CAD build for the part. Positions are in the model's coordinates, mm. A direction names the side the tool comes from. Give positions to 0.01 mm unless a question says otherwise; leave off trailing zeros. Write each loop counter-clockwise with the first axis right and the second up, starting at its lowest first coordinate (ties: lowest second). Pieces come first, ordered by that corner, then holes. Notation, with made-up numbers: (79.25, -39.75) -> (121.25, -39.75) arc R17 cw to (121.25, -34.75) -> close; hole circle Ø4 at (12.25, -4.75). An arc over 180 degrees is marked (long way). Answer as a JSON object with one key per item and string values.
```python
from build123d import *

# Parameters (mm, degrees)
F1_DEPTH  = 20
F3_R      = 3.5
F4_DEPTH  = 10
F8_R      = 3.5
F9_DEPTH  = 1
F9_FACE_R = 3.5


with BuildPart() as f1:
    # F0 (on Front) → F1 (new body)
    with BuildSketch(Plane.XZ):
        Polygon((0, -40), (0, 0), (60, 0), (60, 5), (-5, 5), (-5, -45), (40, -45), (40, -40), align=None)
    extrude(amount=F1_DEPTH)

    # F3 (on offset) → F4 (join)
    with BuildSketch(Plane(origin=(0, 0, -45), x_dir=(1, 0, 0), z_dir=(0, 0, -1))):
        with Locations((33.4731638432, 10)):
            Circle(F3_R)
    extrude(amount=F4_DEPTH)



with BuildPart() as f9:
    # F8 (on offset) → F9 (new body)
    with BuildSketch(Plane(origin=(0, 0, -55), x_dir=(1, 0, 0), z_dir=(0, 0, -1))):
        with Locations((13.4731638432, 10)):
            Circle(F8_R)
    extrude(amount=-F9_DEPTH)


with BuildPart() as f1_1:
    add(f1.part)

    add(f9.part)  # F10 merges F9
    # F10: sweep along a path in F6
    with BuildLine(Plane(origin=(0, -10, 0), x_dir=(-1, 0, 0), z_dir=(0, 1, 0))) as f10_path:
        ThreePointArc((-33.4731638432, -55), (-23.4731638432, -65), (-13.4731638432, -55))
    # F9_face (on face) → F10 (sweep)
    with BuildSketch(Plane(origin=(13.4731638432, -10, -55), x_dir=(1, 0, 0), z_dir=(0, 0, -1))):
        Circle(F9_FACE_R)
    sweep(path=f10_path.line)


solid = f1_1.part
```
1) Slice it at C-C (z = -38.5). List the corners of the cut face in (x, y).
Model answer:
{"outline": "(-5, -20) -> (0, -20) -> (0, 0) -> (-5, 0) -> close"}
2) Pin check, flat tip, straight feed: pin 1 (2.5 mm diameter, centred on y = -9, z = -41.5, fed in from +X). Stop position of the tip, or through.
Model answer:
{"pin 1": "stops at x = 40"}
3) Wall check: probe 1 along Z at (x, y) = (7, -11.5); probe 2 along Z at (x, y) = (22, -7.25); probe 3 along Z at (x, y) = (45.5, -12). Give the ranges that are in metal, low to high.
Model answer:
{"probe 1": "z = -45 to -40, 0 to 5", "probe 2": "z = -67.08 to -62.7, -45 to -40, 0 to 5", "probe 3": "z = 0 to 5"}
4) Slice it at B-B (x = 29). State how many separate pieces and enclosed holes the cut face has, then the cut area to 3 significant figures.
Model answer:
{"separate pieces": "3", "enclosed holes": "0", "area": "248 mm2"}
5) Slice it at D-D (y = -10). List the corners of the cut face in (x, z), then the cut area to 3 significant figures.
Model answer:
{"outline": "(-5, -45) -> (29.97, -45) -> (29.97, -55) arc R6.5 cw to (16.97, -55) -> (16.97, -54) -> (9.97, -54) -> (9.97, -55) arc R13.5 ccw to (36.97, -55) -> (36.97, -45) -> (40, -45) -> (40, -40) -> (0, -40) -> (0, 0) -> (60, 0) -> (60, 5) -> (-5, 5) -> close", "area": "1,050 mm2"}
6) 3-axis set-ups, long thin cutter, end or side, ignore diameter. For faces 4 (the cylindrical face through (12.714, -6.583, -54.507)), 5 (the flat face through (13, -10, -54)), 6 (the flat face through (30, -10, 0)), 7 (the flat face through (40, -10, -43)): which of +Z, -Z, +X, -X, +Y, -Y reach the whole face in a straight line?
Model answer:
{"face 4": "none", "face 5": "-X, +Y, -Y", "face 6": "+X, +Y, -Y", "face 7": "-Z, +X, +Y, -Y"}
7) Slice it at A-A (y = -14.5). List the corners of the cut face in (x, z).
Model answer:
{"outline": "(-5, -45) -> (40, -45) -> (40, -40) -> (0, -40) -> (0, 0) -> (60, 0) -> (60, 5) -> (-5, 5) -> close"}
8) Mould opens along Z. For faces 1 (the flat face through (28, -10, 5)), 2 (the flat face through (17, -10, -45)), 3 (the flat face through (60, -10, 2)) say: released by +Z, released by -Z, zero draft, split by the parting line, or undercut.
Model answer:
{"face 1": "released by +Z", "face 2": "undercut", "face 3": "zero draft"}
